Part model, mm, in its own coordinate system. Face numbers are marked on the shaded views. A direction names the side the tool comes from. Give positions to 0.01 mm unless a question says otherwise; leave off trailing zeros. Loops run counter-clockwise (first coordinate to the right, second up) from the corner with the lowest first, then second, coordinate; pieces in that order, holes last. Notation, with made-up numbers: (-30.75, -25.75) -> (-19.75, -25.75) arc R36 ccw to (-19.75, 10.25) -> close; hole circle Ø2 at (10, 31). An arc over 180 degrees is marked (long way). One line per question, with ' | ' between items.
```python
from build123d import *

# Parameters (mm, degrees)
SKETCH_2_W          = 10
SKETCH_2_H          = 18
EXTRUDE_1_DEPTH     = 3
SKETCH_3_R          = 2.5
CUT_EXTRUDE_1_DEPTH = 21.808652047
FILLET_1_R          = 5
SKETCH_4_W          = 10
SKETCH_4_H          = 3
EXTRUDE_2_DEPTH     = 15
FILLET_2_R          = 5
SKETCH_5_R          = 2.5
CUT_EXTRUDE_2_DEPTH = 26.475478406
SKETCH_6_R          = 2.5
EXTRUDE_3_DEPTH     = 3
SKETCH_7_R          = 2.5
CUT_EXTRUDE_3_DEPTH = 26.475478406
SKETCH_8_R          = 2.580933604
EXTRUDE_4_DEPTH     = 3
SKETCH_9_R          = 2.5
CUT_EXTRUDE_4_DEPTH = 26.475478406
SKETCH_10_R         = 2.5
EXTRUDE_5_DEPTH     = 3
SKETCH_11_R         = 2.5
CUT_EXTRUDE_5_DEPTH = 26.475478406


with BuildPart() as part:
    # 草图2 → 凸台-拉伸1 (new body)
    with BuildSketch(Plane.XY):
        with Locations((5, -9)):
            Rectangle(SKETCH_2_W, SKETCH_2_H)
    extrude(amount=EXTRUDE_1_DEPTH)

    # 草图3 → 切除-拉伸1 (cut, through all)
    with BuildSketch(Plane.XY.offset(3)):
        with Locations((5, -9.74)):
            Circle(SKETCH_3_R)
    extrude(amount=-CUT_EXTRUDE_1_DEPTH, mode=Mode.SUBTRACT)

    # 圆角1
    fillet_1_edges = [part.edges().sort_by_distance(p)[0] for p in [
        (10, -18, 1.5),
        (0, -18, 1.5),
    ]]
    fillet(fillet_1_edges, radius=FILLET_1_R - 0.0001)  # a hair under: the kernel refuses the full size

    # 草图4 → 凸台-拉伸2 (add)
    with BuildSketch(Plane.XY.offset(3)):
        with Locations((5, -1.5)):
            Rectangle(SKETCH_4_W, SKETCH_4_H)
    extrude(amount=EXTRUDE_2_DEPTH)

    # 圆角2
    fillet_2_edges = [part.edges().sort_by_distance(p)[0] for p in [
        (10, -1.5, 18),
        (0, -1.5, 18),
    ]]
    fillet(fillet_2_edges, radius=FILLET_2_R - 0.0001)  # a hair under: the kernel refuses the full size

    # 草图5 → 切除-拉伸2 (cut, through all)
    with BuildSketch(Plane.XZ.offset(3)):
        with Locations(Location((5, 11.11, 0), (0, 0, 270))):
            Circle(SKETCH_5_R)
    extrude(amount=-CUT_EXTRUDE_2_DEPTH, mode=Mode.SUBTRACT)

    # 草图6 → 凸台-拉伸3 (add)
    with BuildSketch(Plane.XZ.offset(3)):
        with Locations((5, 11.11)):
            Circle(SKETCH_6_R)
    extrude(amount=-EXTRUDE_3_DEPTH)

    # 草图7 → 切除-拉伸3 (cut, through all)
    with BuildSketch(Plane(origin=(0, -3, 0), x_dir=(-1, 0, 0), z_dir=(0, -1, 0))):
        with Locations(Location((-5, -12.02, 0), (0, 0, 90))):
            Circle(SKETCH_7_R)
    extrude(amount=-CUT_EXTRUDE_3_DEPTH, mode=Mode.SUBTRACT)

    # 草图8 → 凸台-拉伸4 (add)
    with BuildSketch(Plane.XZ.offset(3)):
        with Locations((5, 12.02)):
            Circle(SKETCH_8_R)
    extrude(amount=-EXTRUDE_4_DEPTH)

    # 草图9 → 切除-拉伸4 (cut, through all)
    with BuildSketch(Plane.XZ.offset(3)):
        with Locations(Location((5, 8.11, 0), (0, 0, 270))):
            Circle(SKETCH_9_R)
    extrude(amount=-CUT_EXTRUDE_4_DEPTH, mode=Mode.SUBTRACT)

    # 草图10 → 凸台-拉伸5 (add)
    with BuildSketch(Plane.XZ.offset(3)):
        with Locations((5, 8.11)):
            Circle(SKETCH_10_R)
    extrude(amount=-EXTRUDE_5_DEPTH)

    # 草图11 → 切除-拉伸5 (cut, through all)
    with BuildSketch(Plane.XZ.offset(3)):
        with Locations(Location((5, 9.74, 0), (0, 0, 270))):
            Circle(SKETCH_11_R)
    extrude(amount=-CUT_EXTRUDE_5_DEPTH, mode=Mode.SUBTRACT)


solid = part.part
```
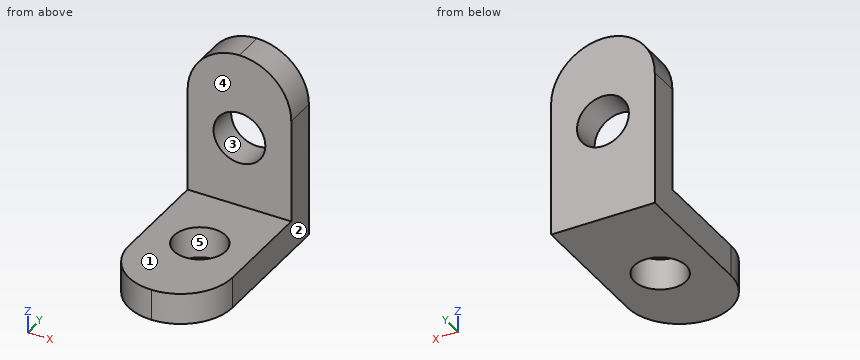
1) Drill centre lines: line 1 (X direction, y = -1.25, z = 9.74); line 2 (Z direction, x = 6, y = -16.75); line 3 (Y direction, x = 5, z = 1.1). Where is each one in solid material? Low to high.
Found:
line 1: 0 to 2.5, 7.5 to 10 | line 2: 0 to 3 | line 3: -18 to -12.24, -7.24 to 0
2) Saw through at B-B (z = 9.74). Give the cut face in (x, y), and give its area (3 significant figures).
Found:
outline: (0, -3) -> (2.5, -3) -> (2.5, 0) -> (0, 0) -> close; (7.5, -3) -> (10, -3) -> (10, 0) -> (7.5, 0) -> close | area: 15.0 mm2
3) Saw through at A-A (y = -9.74). Give the cut face in (x, z).
Found:
outline: (0, 0) -> (2.5, 0) -> (2.5, 3) -> (0, 3) -> close; (7.5, 0) -> (10, 0) -> (10, 3) -> (7.5, 3) -> close
4) Saw through at D-D (x = 6.5). Give the cut face in (y, z).
Found:
outline: (-17.77, 0) -> (-11.74, 0) -> (-11.74, 3) -> (-17.77, 3) -> close; (-7.74, 0) -> (0, 0) -> (0, 7.74) -> (-3, 7.74) -> (-3, 3) -> (-7.74, 3) -> close; (-3, 11.74) -> (0, 11.74) -> (0, 17.77) -> (-3, 17.77) -> close
5) Tool access for the marked faces 4 and 5: list every direction of +Z, -Z, +X, -X, +Y, -Y with a clear straight run to the whole face (end or side of a thin tool).
Found:
face 4: +Z, +X, -X, -Y | face 5: +Z, -Z
6) Pull direction X, two halves, no side cores. Call the marked faces 1, 2 and 3: pulls with the +X half, pulls with the -X half, needs draft (parallel to the pull), parting line crosses it, or undercut.
Found:
face 1: needs draft | face 2: pulls with the +X half | face 3: undercut
7) Pin check, flat tip, straight feed: P1, Ø5, axis at x = 4, z = 7, coming from the -Y side. Stop position of the tip, or through.
Found:
P1: y = -3
